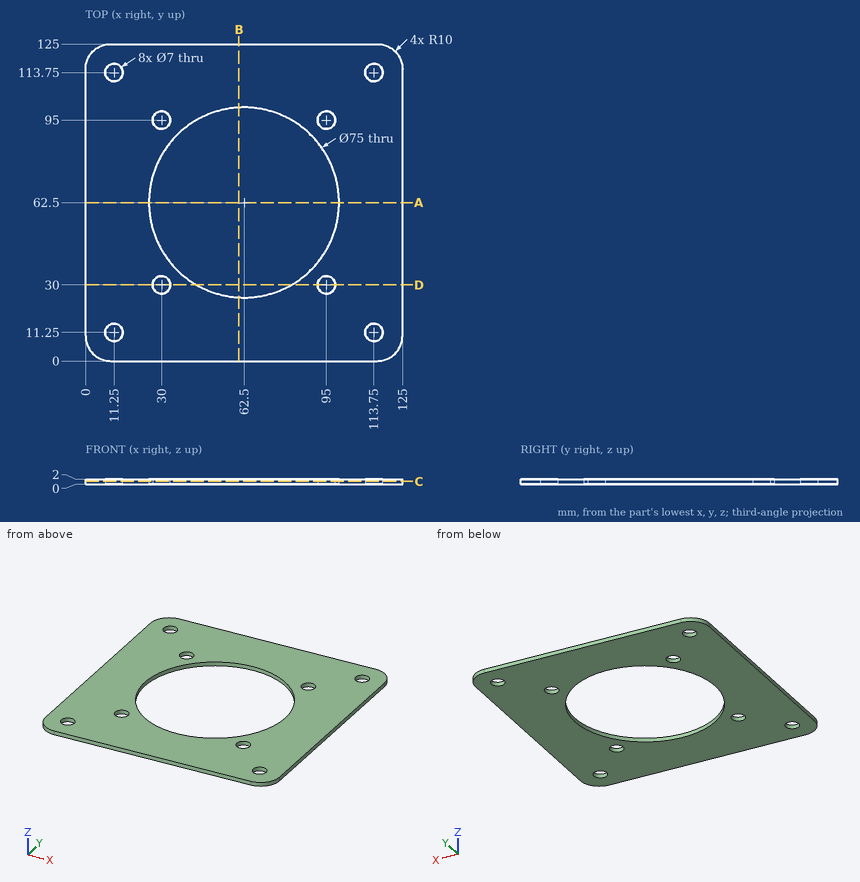
Print and shaded views of the part. All mm, measured from the part's lowest x, y and z. Coordinates: 2 decimals unless noted, no trailing zeros. Loops run counter-clockwise (first coordinate to the right, second up) from the corner with the lowest first, then second, coordinate; pieces in that order, holes last. Notation, with made-up numbers: (-17.5, 72.25) -> (21.5, 72.25) arc R21 cw to (21.5, 93.25) -> close; hole circle Ø6 at (46.25, 64). An arc over 180 degrees is marked (long way). Use one line per item in the form item = value. Start each with the question number.
(1) Flat gauge pin, fed straight in: pin 1 (10 mm diameter, centred on x = 102, y = 100, fed in from -Z). Where does the tip first touch, or does it go through?
(2) Cut at A-A on y = 62.5. Give the cut face in (x, z).
(3) Cut at B-B on x = 60.5. Give the cut face in (y, z).
(4) Cut at D-D on y = 30. Give the cut face in (x, z), and give its area (3 significant figures).
(5) Probe probe 1 along X at (y, z) = (113.75, 1); probe 2 along Y at (x, z) = (11, 1.85); probe 3 along Y at (x, z) = (9, 0.9). List the from-to ranges inside material, lowest first. Write a range as from..to.
(6) Cut at C-C on z = 1.05. Give the number of separate pieces and of enclosed holes in the cut face, and give its area (3 significant figures).
Values:
q1.pin_1 = 0
q2.outline = (0, 0) -> (25, 0) -> (25, 2) -> (0, 2) -> close; (100, 0) -> (125, 0) -> (125, 2) -> (100, 2) -> close
q3.outline = (0, 0) -> (25.05, 0) -> (25.05, 2) -> (0, 2) -> close; (99.95, 0) -> (125, 0) -> (125, 2) -> (99.95, 2) -> close
q4.outline = (0, 0) -> (26.5, 0) -> (26.5, 2) -> (0, 2) -> close; (33.5, 0) -> (43.79, 0) -> (43.79, 2) -> (33.5, 2) -> close; (81.21, 0) -> (91.5, 0) -> (91.5, 2) -> (81.21, 2) -> close; (98.5, 0) -> (125, 0) -> (125, 2) -> (98.5, 2) -> close
q4.area = 147 mm2
q5.probe_1 = 0..7.75, 14.75..110.25, 117.25..125
q5.probe_2 = 0..7.76, 14.74..110.26, 117.24..125
q5.probe_3 = 0.05..8.57, 13.93..111.07, 116.43..124.95
q6.separate_pieces = 1
q6.enclosed_holes = 9
q6.area = 10,800 mm2
